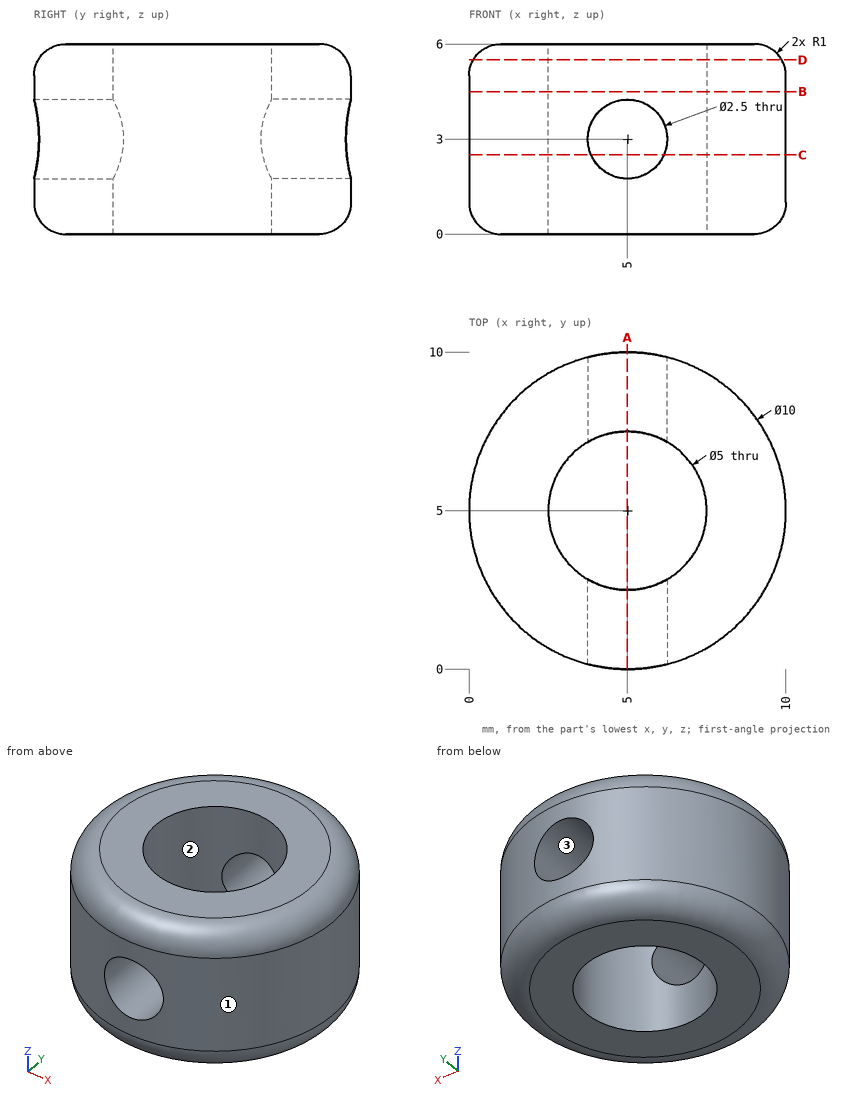
Print and shaded views of the part. All mm, measured from the part's lowest x, y and z. Coordinates: 2 decimals unless noted, no trailing zeros. Order: outer loops, then holes, each group sorted by start corner. A loop starts at its lowest first (then second) coordinate and runs counter-clockwise, first axis right, second up.
Item 1: Saw through at B-B on z = 4.5. List the corners of the cut face in (x, y).
Filled in:
outline: circle Ø10 at (5, 5); hole circle Ø5 at (5, 5)
Item 2: Saw through at A-A on x = 5. State how many separate pieces and enclosed holes the cut face has, then the cut area to 3 significant figures.
Filled in:
separate pieces: 4
enclosed holes: 0
area: 16.6 mm2
Item 3: Saw through at D-D on z = 5.5. List the corners of the cut face in (x, y), then the cut area to 3 significant figures.
Filled in:
outline: circle Ø9.73 at (5, 5); hole circle Ø5 at (5, 5)
area: 54.8 mm2
Item 4: Saw through at C-C on z = 2.5. List the corners of the cut face in (x, y), then the cut area to 3 significant figures.
Filled in:
outline: (3.85, 0.13) - (3.85, 2.78) arc R2.5 cw to (3.85, 7.22) - (3.85, 9.87) arc R5 ccw to start; (6.15, 0.13) arc R5 ccw to (6.15, 9.87) - (6.15, 7.22) arc R2.5 cw to (6.15, 2.78) - close
area: 47.2 mm2
Item 5: Drill centre lines: L1, parallel to Z at x = 5, y = 8.75; L2, parallel to Y at x = 6, z = 4.5; L3, parallel to X at y = 7.75, z = 2.75. Where is each one in solid material? Low to high.
Filled in:
L1: z = 0 to 1.75, 4.25 to 6
L2: y = 0.1 to 2.71, 7.29 to 9.9
L3: x = 0.82 to 3.78, 6.22 to 9.18
Item 6: Mould opens along Y. For the marked faces 1, 2 and 3 say: released by +Y, released by -Y, zero draft, split by the parting line, or undercut.
Filled in:
face 1: split by the parting line
face 2: undercut
face 3: zero draft
Item 7: Drop flat-ended pins along their axis: pin 1 Ø1.5 at (x, z) = (6.5, 3) entering from +Y; pin 2 Ø1 at (y, z) = (7, 2.5) entering from +X; pin 3 Ø1 at (x, z) = (8.5, 3) entering from -Y. Give the stop position or say it passes through.
Filled in:
pin 1: stops at y = 9.88
pin 2: stops at x = 9.77
pin 3: stops at y = 1
